from build123d import *

# Parameters (mm, degrees)
SKETCH1_R                    = 2.5
SKETCH1_R_2                  = 1.8
SKETCH1_R_3                  = 2.55
SKETCH1_R_4                  = 11.05
BOSS_EXTRUDE1_DEPTH          = 1.6
SKETCHED_START               = -26.738102053
SKETCHED_BEND1_OUTLINE_W     = 83
SKETCHED_BEND1_OUTLINE_H     = 1.6
SKETCHED_BEND1_DEPTH         = 45.741537679
SKETCHED_START_2             = 42.203435626
SKETCHED_BEND1_2_OUTLINE_W   = 83
SKETCHED_BEND1_2_OUTLINE_H   = 1.6
SKETCHED_BEND1_2_DEPTH       = 45.741537678
SKETCHED_START_3             = 19.003435626
SKETCHED_BEND1_3_OUTLINE_R   = 2.5
SKETCHED_BEND1_3_OUTLINE_R_2 = 1.8
SKETCHED_BEND1_3_OUTLINE_R_3 = 11.05
SKETCHED_BEND1_3_DEPTH       = 1.6
SKETCHED_START_4             = 40.603435626
SKETCHED_BEND1_4_OUTLINE_R   = 2.5
SKETCHED_BEND1_4_OUTLINE_R_2 = 1.8
SKETCHED_BEND1_4_OUTLINE_R_3 = 11.05
SKETCHED_BEND1_4_DEPTH       = 1.6
SKETCHED_START_5             = -92
SKETCHED_BEND1_5_DEPTH       = 78


with BuildPart() as part:
    # Sketch1 → Boss-Extrude1 (new body)
    with BuildSketch(Plane.XY):
        with BuildLine():
            Line((-91.108168831, 42.903435626), (-91.108168831, 18.303435626))
            ThreePointArc((-91.108168831, 18.303435626), (-93.724463922, 17.219730716), (-94.808168831, 14.603435626))
            Line((-94.808168831, 14.603435626), (-94.808168831, -18.079639731))
            ThreePointArc((-94.808168831, -18.079639731), (-93.724463922, -20.695934821), (-91.108168831, -21.779639731))
            Line((-91.108168831, -21.779639731), (-58.808168831, -21.779639731))
            Line((-58.808168831, -21.779639731), (-58.808168831, -23.038102053))
            ThreePointArc((-58.808168831, -23.038102053), (-57.724463922, -25.654397143), (-55.108168831, -26.738102053))
            Line((-55.108168831, -26.738102053), (-15.508168831, -26.738102053))
            ThreePointArc((-15.508168831, -26.738102053), (-12.891873741, -25.654397143), (-11.808168831, -23.038102053))
            Line((-11.808168831, -23.038102053), (-11.808168831, 14.636324152))
            ThreePointArc((-11.808168831, 14.636324152), (-12.723275427, 17.072380131), (-15.015935712, 18.303435626))
            Line((-15.015935712, 18.303435626), (-15.015935712, 42.903435626))
            ThreePointArc((-15.015935712, 42.903435626), (-12.723275427, 44.13449112), (-11.808168831, 46.570547099))
            Line((-11.808168831, 46.570547099), (-11.808168831, 84.244973304))
            ThreePointArc((-11.808168831, 84.244973304), (-12.891873741, 86.861268394), (-15.508168831, 87.944973304))
            Line((-15.508168831, 87.944973304), (-55.108168831, 87.944973304))
            ThreePointArc((-55.108168831, 87.944973304), (-57.724463922, 86.861268394), (-58.808168831, 84.244973304))
            Line((-58.808168831, 84.244973304), (-58.808168831, 82.986510982))
            Line((-58.808168831, 82.986510982), (-91.108168831, 82.986510982))
            ThreePointArc((-91.108168831, 82.986510982), (-93.724463922, 81.902806072), (-94.808168831, 79.286510982))
            Line((-94.808168831, 79.286510982), (-94.808168831, 46.603435626))
            ThreePointArc((-94.808168831, 46.603435626), (-93.724463922, 43.987140535), (-91.108168831, 42.903435626))
        make_face()
        with Locations((-66.308168831, 72.944973304)):
            Circle(SKETCH1_R, mode=Mode.SUBTRACT)
        with Locations((-50.808168831, 78.444973304)):
            Circle(SKETCH1_R_2, mode=Mode.SUBTRACT)
        with Locations(Location((-19.808168831, 78.444973304, 0), (0, 0, 180))):
            Circle(SKETCH1_R_2, mode=Mode.SUBTRACT)
        with Locations((-19.808168831, 47.444973304)):
            Circle(SKETCH1_R_2, mode=Mode.SUBTRACT)
        with Locations(Location((-50.808168831, 47.444973304, 0), (0, 0, 180))):
            Circle(SKETCH1_R_2, mode=Mode.SUBTRACT)
        with Locations((-86.308168831, 72.944973304)):
            Circle(SKETCH1_R, mode=Mode.SUBTRACT)
        with Locations((-66.308168831, 62.944973304)):
            Circle(SKETCH1_R, mode=Mode.SUBTRACT)
        with Locations((-66.308168831, 52.944973304)):
            Circle(SKETCH1_R, mode=Mode.SUBTRACT)
        with Locations((-86.308168831, 62.944973304)):
            Circle(SKETCH1_R, mode=Mode.SUBTRACT)
        with Locations((-53.062052272, 30.603435626)):
            Circle(SKETCH1_R_3, mode=Mode.SUBTRACT)
        with Locations((-43.062052272, 30.603435626)):
            Circle(SKETCH1_R_3, mode=Mode.SUBTRACT)
        with Locations((-33.062052272, 30.603435626)):
            Circle(SKETCH1_R_3, mode=Mode.SUBTRACT)
        with Locations((-23.062052272, 30.603435626)):
            Circle(SKETCH1_R_3, mode=Mode.SUBTRACT)
        with Locations((-63.062052272, 30.603435626)):
            Circle(SKETCH1_R_3, mode=Mode.SUBTRACT)
        with Locations((-73.062052272, 30.603435626)):
            Circle(SKETCH1_R_3, mode=Mode.SUBTRACT)
        with Locations((-83.062052272, 30.603435626)):
            Circle(SKETCH1_R_3, mode=Mode.SUBTRACT)
        with Locations((-35.308168831, 62.944973304)):
            Circle(SKETCH1_R_4, mode=Mode.SUBTRACT)
        with Locations((-86.308168831, 52.944973304)):
            Circle(SKETCH1_R, mode=Mode.SUBTRACT)
        with Locations(Location((-35.308168831, -1.738102053, 0), (0, 0, 180))):
            Circle(SKETCH1_R_4, mode=Mode.SUBTRACT)
        with Locations((-19.808168831, -17.238102053)):
            Circle(SKETCH1_R_2, mode=Mode.SUBTRACT)
        with Locations(Location((-19.808168831, 13.761897947, 0), (0, 0, 180))):
            Circle(SKETCH1_R_2, mode=Mode.SUBTRACT)
        with Locations((-50.808168831, 13.761897947)):
            Circle(SKETCH1_R_2, mode=Mode.SUBTRACT)
        with Locations(Location((-50.808168831, -17.238102053, 0), (0, 0, 180))):
            Circle(SKETCH1_R_2, mode=Mode.SUBTRACT)
        with Locations(Location((-66.308168831, -11.738102053, 0), (0, 0, 180))):
            Circle(SKETCH1_R, mode=Mode.SUBTRACT)
        with Locations(Location((-66.308168831, -1.738102053, 0), (0, 0, 180))):
            Circle(SKETCH1_R, mode=Mode.SUBTRACT)
        with Locations(Location((-66.308168831, 8.261897947, 0), (0, 0, 180))):
            Circle(SKETCH1_R, mode=Mode.SUBTRACT)
        with Locations(Location((-86.308168831, 8.261897947, 0), (0, 0, 180))):
            Circle(SKETCH1_R, mode=Mode.SUBTRACT)
        with Locations(Location((-86.308168831, -1.738102053, 0), (0, 0, 180))):
            Circle(SKETCH1_R, mode=Mode.SUBTRACT)
        with Locations(Location((-86.308168831, -11.738102053, 0), (0, 0, 180))):
            Circle(SKETCH1_R, mode=Mode.SUBTRACT)
    extrude(amount=BOSS_EXTRUDE1_DEPTH)

    # Sketched Bend1: read off the stored shape, not the designer's step
    # Sketched Bend1 outline → Sketched Bend1 (cut)
    with BuildSketch(Plane(origin=(0, 0, 0), x_dir=(1, 0, 0), z_dir=(0, 1, 0)).offset(SKETCHED_START)):
        with Locations((-53.308168831, -0.8)):
            Rectangle(SKETCHED_BEND1_OUTLINE_W, SKETCHED_BEND1_OUTLINE_H)
    extrude(amount=SKETCHED_BEND1_DEPTH, mode=Mode.SUBTRACT)

    # Sketched Bend1 2 outline → Sketched Bend1 2 (cut)
    with BuildSketch(Plane(origin=(0, 0, 0), x_dir=(1, 0, 0), z_dir=(0, 1, 0)).offset(SKETCHED_START_2)):
        with Locations((-53.308168831, -0.8)):
            Rectangle(SKETCHED_BEND1_2_OUTLINE_W, SKETCHED_BEND1_2_OUTLINE_H)
    extrude(amount=SKETCHED_BEND1_2_DEPTH, mode=Mode.SUBTRACT)

    # Sketched Bend1 3 outline → Sketched Bend1 3 (add)
    with BuildSketch(Plane(origin=(0, 0, 0), x_dir=(1, 0, 0), z_dir=(0, 1, 0)).offset(SKETCHED_START_3)):
        with BuildLine():
            Line((-15.015935712, -2.643362939), (-15.015935712, -1.6))
            Line((-15.015935712, -1.6), (-91.108168831, -1.6))
            Line((-91.108168831, -1.6), (-91.108168831, -2.643362939))
            ThreePointArc((-91.108168831, -2.643362939), (-93.724463922, -3.727067848), (-94.808168831, -6.343362939))
            Line((-94.808168831, -6.343362939), (-94.808168831, -39.026438295))
            ThreePointArc((-94.808168831, -39.026438295), (-93.724463922, -41.642733385), (-91.108168831, -42.726438295))
            Line((-91.108168831, -42.726438295), (-58.808168831, -42.726438295))
            Line((-58.808168831, -42.726438295), (-58.808168831, -43.984900617))
            ThreePointArc((-58.808168831, -43.984900617), (-57.724463922, -46.601195708), (-55.108168831, -47.684900617))
            Line((-55.108168831, -47.684900617), (-15.508168831, -47.684900617))
            ThreePointArc((-15.508168831, -47.684900617), (-12.891873741, -46.601195707), (-11.808168831, -43.984900617))
            Line((-11.808168831, -43.984900617), (-11.808168831, -6.310474412))
            ThreePointArc((-11.808168831, -6.310474412), (-12.723275427, -3.874418433), (-15.015935712, -2.643362939))
        make_face()
        with Locations((-86.308168831, -32.684900617)):
            Circle(SKETCHED_BEND1_3_OUTLINE_R, mode=Mode.SUBTRACT)
        with Locations((-66.308168831, -32.684900617)):
            Circle(SKETCHED_BEND1_3_OUTLINE_R, mode=Mode.SUBTRACT)
        with Locations((-50.808168831, -38.184900617)):
            Circle(SKETCHED_BEND1_3_OUTLINE_R_2, mode=Mode.SUBTRACT)
        with Locations((-19.808168831, -38.184900617)):
            Circle(SKETCHED_BEND1_3_OUTLINE_R_2, mode=Mode.SUBTRACT)
        with Locations((-86.308168831, -22.684900617)):
            Circle(SKETCHED_BEND1_3_OUTLINE_R, mode=Mode.SUBTRACT)
        with Locations((-86.308168831, -12.684900617)):
            Circle(SKETCHED_BEND1_3_OUTLINE_R, mode=Mode.SUBTRACT)
        with Locations((-66.308168831, -22.684900617)):
            Circle(SKETCHED_BEND1_3_OUTLINE_R, mode=Mode.SUBTRACT)
        with Locations((-66.308168831, -12.684900617)):
            Circle(SKETCHED_BEND1_3_OUTLINE_R, mode=Mode.SUBTRACT)
        with Locations((-35.308168831, -22.684900617)):
            Circle(SKETCHED_BEND1_3_OUTLINE_R_3, mode=Mode.SUBTRACT)
        with Locations((-50.808168831, -7.184900617)):
            Circle(SKETCHED_BEND1_3_OUTLINE_R_2, mode=Mode.SUBTRACT)
        with Locations((-19.808168831, -7.184900617)):
            Circle(SKETCHED_BEND1_3_OUTLINE_R_2, mode=Mode.SUBTRACT)
    extrude(amount=SKETCHED_BEND1_3_DEPTH)

    # Sketched Bend1 4 outline → Sketched Bend1 4 (add)
    with BuildSketch(Plane(origin=(0, 0, 0), x_dir=(1, 0, 0), z_dir=(0, 1, 0)).offset(SKETCHED_START_4)):
        with BuildLine():
            Line((-15.015935712, -2.643362939), (-15.015935712, -1.6))
            Line((-15.015935712, -1.6), (-91.108168831, -1.6))
            Line((-91.108168831, -1.6), (-91.108168831, -2.643362939))
            ThreePointArc((-91.108168831, -2.643362939), (-93.724463922, -3.727067848), (-94.808168831, -6.343362939))
            Line((-94.808168831, -6.343362939), (-94.808168831, -39.026438295))
            ThreePointArc((-94.808168831, -39.026438295), (-93.724463922, -41.642733385), (-91.108168831, -42.726438295))
            Line((-91.108168831, -42.726438295), (-58.808168831, -42.726438295))
            Line((-58.808168831, -42.726438295), (-58.808168831, -43.984900617))
            ThreePointArc((-58.808168831, -43.984900617), (-57.724463922, -46.601195708), (-55.108168831, -47.684900617))
            Line((-55.108168831, -47.684900617), (-15.508168831, -47.684900617))
            ThreePointArc((-15.508168831, -47.684900617), (-12.891873741, -46.601195707), (-11.808168831, -43.984900617))
            Line((-11.808168831, -43.984900617), (-11.808168831, -6.310474412))
            ThreePointArc((-11.808168831, -6.310474412), (-12.723275427, -3.874418433), (-15.015935712, -2.643362939))
        make_face()
        with Locations((-86.308168831, -32.684900617)):
            Circle(SKETCHED_BEND1_4_OUTLINE_R, mode=Mode.SUBTRACT)
        with Locations((-66.308168831, -32.684900617)):
            Circle(SKETCHED_BEND1_4_OUTLINE_R, mode=Mode.SUBTRACT)
        with Locations((-50.808168831, -38.184900617)):
            Circle(SKETCHED_BEND1_4_OUTLINE_R_2, mode=Mode.SUBTRACT)
        with Locations((-19.808168831, -38.184900617)):
            Circle(SKETCHED_BEND1_4_OUTLINE_R_2, mode=Mode.SUBTRACT)
        with Locations((-86.308168831, -22.684900617)):
            Circle(SKETCHED_BEND1_4_OUTLINE_R, mode=Mode.SUBTRACT)
        with Locations((-86.308168831, -12.684900617)):
            Circle(SKETCHED_BEND1_4_OUTLINE_R, mode=Mode.SUBTRACT)
        with Locations((-66.308168831, -22.684900617)):
            Circle(SKETCHED_BEND1_4_OUTLINE_R, mode=Mode.SUBTRACT)
        with Locations((-66.308168831, -12.684900617)):
            Circle(SKETCHED_BEND1_4_OUTLINE_R, mode=Mode.SUBTRACT)
        with Locations((-35.308168831, -22.684900617)):
            Circle(SKETCHED_BEND1_4_OUTLINE_R_3, mode=Mode.SUBTRACT)
        with Locations((-50.808168831, -7.184900617)):
            Circle(SKETCHED_BEND1_4_OUTLINE_R_2, mode=Mode.SUBTRACT)
        with Locations((-19.808168831, -7.184900617)):
            Circle(SKETCHED_BEND1_4_OUTLINE_R_2, mode=Mode.SUBTRACT)
    extrude(amount=SKETCHED_BEND1_4_DEPTH)

    # Sketched Bend1 5 outline → Sketched Bend1 5 (cut)
    with BuildSketch(Plane.YZ.offset(SKETCHED_START_5)):
        with BuildLine():
            Line((42.203435626, 0), (42.203435626, 1.6))
            ThreePointArc((42.203435626, 1.6), (41.734806476, 0.46862915), (40.603435626, 0))
            Line((40.603435626, 0), (42.203435626, 0))
        make_face()
        with BuildLine():
            Line((19.003435626, 0), (20.603435626, 0))
            ThreePointArc((20.603435626, 0), (19.472064776, 0.46862915), (19.003435626, 1.6))
            Line((19.003435626, 1.6), (19.003435626, 0))
        make_face()
    extrude(amount=SKETCHED_BEND1_5_DEPTH, mode=Mode.SUBTRACT)


solid = part.part
Geometry: final body of the model. Coordinates: model frame, mm. A direction names the side the tool comes from. Coordinates: 2 decimals unless noted, no trailing zeros. Order: outer loops, then holes, each group sorted by start corner. A loop starts at its lowest first (then second) coordinate and runs counter-clockwise, first axis right, second up.
(1) Draft query along X for faces 3 (the face through (-68.806, 19.792, 12.575)), 4 (the face through (-94.808, 41, 22)), 5 (the face through (-36, 41, 47.685)). Return one class per face: pulls with the +X half, pulls with the -X half, needs draft (parallel to the pull), parting line crosses it, or undercut.
(2) Access query for faces 1 (the face through (-20.04, 19.79, 36.4)), 2 (the face through (-91.108, 30, 1)). Directions: +Z, -Z, +X, -X, +Y, -Y. A direction counts if a zero-diameter tool reaches every point of the face in a straight line with its end or side. Return the directions, or none.
(3) Section query C-C (z = 19). Return the cut outline in (x, y), plus the area to 3 significant figures.
(4) Section query A-A (x = -42). Return the cut outline in (y, z).
(5) Section query D-D (x = -29.5). Return the cut outline in (y, z), plus the area to 3 significant figures.
(6) First-contact query: pin 1 (1.3 mm diameter, centred on x = -77.5, y = 41.5, fed in from +Z); pin 2 (8 mm diameter, centred on x = -43.06, y = 30.6, fed in from +Z); pin 3 (1.3 mm diameter, centred on y = 26.5, z = 0.5, fed in from -X). Flat tips, straight axial feed; report the tip coordinate or a pass-through.
(7) Material intervals for probe 1 along Y at (x, z) = (-17.5, 4); probe 2 along Z at (x, y) = (-19, 40.75); probe 3 along Z at (x, y) = (-39.5, 33), sorted ascending.
(8) Section query B-B (y = 32.25). State how many separate pieces and enclosed holes the cut face has, plus the area to 3 significant figures.
Solution:
1. face 3: undercut
1. face 4: pulls with the -X half
1. face 5: needs draft
2. face 1: +Y, -Y
2. face 2: -Z, -X, +Y, -Y
3. outline: (-94.81, 19) - (-45.73, 19) - (-45.73, 20.6) - (-94.81, 20.6) - close; (-94.81, 40.6) - (-45.73, 40.6) - (-45.73, 42.2) - (-94.81, 42.2) - close; (-24.89, 19) - (-11.81, 19) - (-11.81, 20.6) - (-24.89, 20.6) - close; (-24.89, 40.6) - (-11.81, 40.6) - (-11.81, 42.2) - (-24.89, 42.2) - close
3. area: 199 mm2
4. outline: (19, 1.6) arc R1.6 ccw to (20.6, 0) - (28.29, 0) - (28.29, 1.6) - (20.6, 1.6) - (20.6, 13.89) - (19, 13.89) - close; (19, 31.48) - (20.6, 31.48) - (20.6, 47.68) - (19, 47.68) - close; (32.92, 0) - (40.6, 0) arc R1.6 ccw to (42.2, 1.6) - (42.2, 13.89) - (40.6, 13.89) - (40.6, 1.6) - (32.92, 1.6) - close; (40.6, 31.48) - (42.2, 31.48) - (42.2, 47.68) - (40.6, 47.68) - close
5. outline: (19, 1.6) arc R1.6 ccw to (20.6, 0) - (40.6, 0) arc R1.6 ccw to (42.2, 1.6) - (42.2, 13.28) - (40.6, 13.28) - (40.6, 1.6) - (20.6, 1.6) - (20.6, 13.28) - (19, 13.28) - close; (19, 32.09) - (20.6, 32.09) - (20.6, 47.68) - (19, 47.68) - close; (40.6, 32.09) - (42.2, 32.09) - (42.2, 47.68) - (40.6, 47.68) - close
5. area: 123 mm2
6. pin 1: stops at z = 42.73
6. pin 2: stops at z = 1.6
6. pin 3: stops at x = -91.11
7. probe 1: y = 19 to 20.6, 40.6 to 42.2
7. probe 2: z = 0.01 to 5.58, 8.79 to 36.58, 39.79 to 47.68
7. probe 3: z = 0 to 1.6
8. separate pieces: 8
8. enclosed holes: 0
8. area: 78.1 mm2
